Input: dimensioned drawing with shaded views. Units: mm. Origin: part minimum x, y, z. Coordinates: 2 decimals unless noted, no trailing zeros. Order: outer loops, then holes, each group sorted by start corner. A loop starts at its lowest first (then second) coordinate and runs counter-clockwise, first axis right, second up.
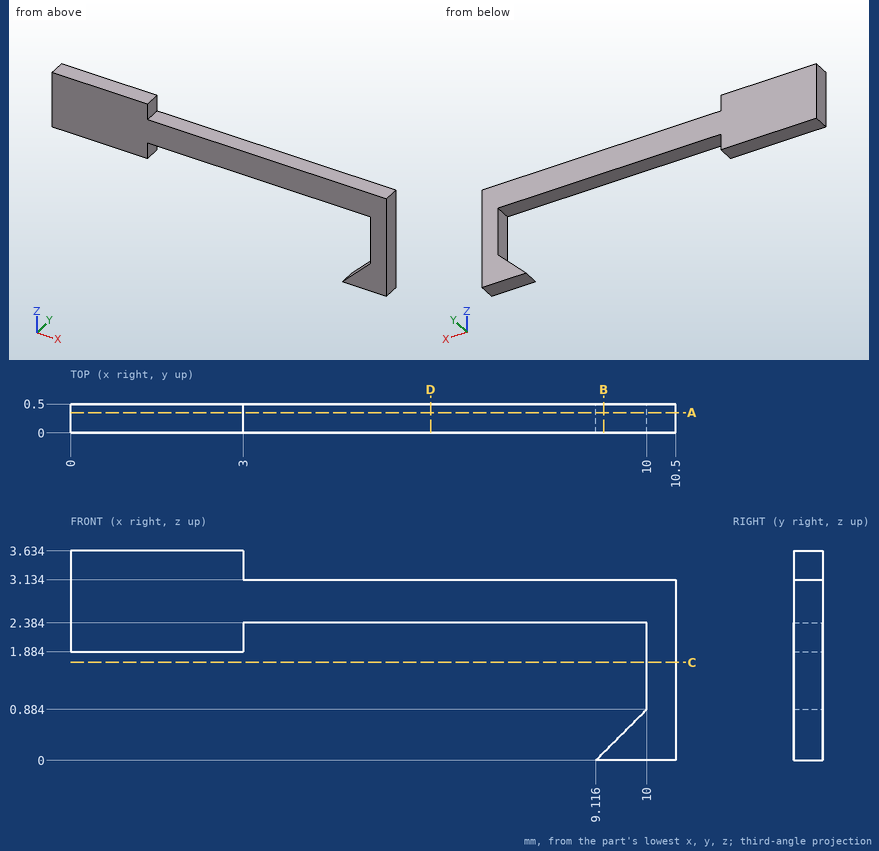
1. Section query B-B on x = 9.25. Return loops of the section in (y, z).
Findings:
outline: (0, 0) - (0.5, 0) - (0.5, 0.13) - (0, 0.13) - close; (0, 2.38) - (0.5, 2.38) - (0.5, 3.13) - (0, 3.13) - close
2. Ray query, line 1 (X direction, y = 0.1, z = 1.05); line 2 (Z direction, x = 7.5, y = 0.25); line 3 (Z direction, x = 2.25, y = 0.3). Return the intervals inside material, ascending.
Findings:
line 1: x = 10 to 10.5
line 2: z = 2.38 to 3.13
line 3: z = 1.88 to 3.63
3. Section query C-C on z = 1.7. Return loops of the section in (x, y), plus the area to 3 significant figures.
Findings:
outline: (10, 0) - (10.5, 0) - (10.5, 0.5) - (10, 0.5) - close
area: 0.250 mm2
4. Section query D-D on x = 6.25. Return loops of the section in (y, z).
Findings:
outline: (0, 2.38) - (0.5, 2.38) - (0.5, 3.13) - (0, 3.13) - close
5. Section query A-A on y = 0.35. Return loops of the section in (x, z).
Findings:
outline: (0, 1.88) - (3, 1.88) - (3, 2.38) - (10, 2.38) - (10, 0.88) - (9.12, 0) - (10.5, 0) - (10.5, 3.13) - (3, 3.13) - (3, 3.63) - (0, 3.63) - close
